```python
from build123d import *

# Parameters (mm, degrees)
F0_R     = 1.984375
F1_DEPTH = 9.525
F3_R     = 3.175
F4_DEPTH = 4.7625
F6_DEPTH = 3.96875


with BuildPart() as f1:
    # F0 (on Front) → F1 (new body)
    with BuildSketch(Plane.XZ):
        Circle(F0_R)
    extrude(amount=F1_DEPTH)

    # F3 (on face) → F4 (join)
    with BuildSketch(Plane.XZ.offset(9.525)):
        Circle(F3_R)
    extrude(amount=F4_DEPTH)

    # F5 (on face) → F6 (cut)
    with BuildSketch(Plane.XZ.offset(14.2875)):
        Polygon((1.984375, 1.145679), (0, 2.291359), (-1.984375, 1.145679), (-1.984375, -1.145679), (0, -2.291359), (1.984375, -1.145679), align=None)
    extrude(amount=-F6_DEPTH, mode=Mode.SUBTRACT)


solid = f1.part
```
Work out the finished part from the listing and answer in its coordinate system (mm). A direction names the side the tool comes from. Round coordinates to 2 decimals unless told otherwise and drop trailing zeros. Write each loop counter-clockwise with the first axis right and the second up, starting at its lowest first coordinate (ties: lowest second). Pieces come first, ordered by that corner, then holes.
1) A cutting plane is placed at C-C on y = -5.75. Determine the outline of the cut face in (x, z), and give its area (3 significant figures).
2) A cutting plane is placed at A-A on z = 0. Determine the outline of the cut face in (x, y) (1 decimal), and give its area (3 significant figures).
3) A cutting plane is placed at B-B on x = 1.75. Determine the outline of the cut face in (y, z) (1 decimal).
4) Which of the six approach directions +Z, -Z, +X, -X, +Y, -Y give full straight-line access (tool end or side, diameter ignored) to faces 4 (the face through (0.978, -12.331, -1.727)), 5 (the face through (1, -9.525, -2)), 6 (the face through (0, 0, 0))?
5) Consider probe 1 along Y at (x, z) = (0.25, -1); probe 2 along X at (y, z) = (-12.75, 0.75); probe 3 along Z at (x, y) = (0.5, -11). Determine where each line is inside the solid, lowest interval first.
6) A cutting plane is placed at D-D on x = -3. Determine the outline of the cut face in (y, z) (1 decimal), and give its area (3 significant figures).
7) Determine the mould class of faces 1 (the face through (1.984, -12, 0)), 2 (the face through (1, -14.288, -2)), 3 (the face through (-0.69, -11.87, -3.1)) for opening direction Z: pulls with the +Z half, pulls with the -Z half, needs draft (parallel to the pull), parting line crosses it, or undercut.
8) Flat-ended cylindrical pins translate along their axes: P1, Ø2, axis at y = -6, z = -0.5, coming from the -X side; P2, Ø1.5, axis at y = -2.5, z = 2, coming from the -X side; P3, Ø2, axis at x = -1.5, y = -4, coming from the -Z side; P4, Ø2, axis at x = -1.5, z = 0, coming from the -Y side. Find the tip coordinate at first contact, or state that the pin passes through.
Entries:
1. outline: circle Ø3.97 at (0, 0)
1. area: 12.4 mm2
2. outline: (-3.2, -14.3) - (-2, -14.3) - (-2, -10.3) - (2, -10.3) - (2, -14.3) - (3.2, -14.3) - (3.2, -9.5) - (2, -9.5) - (2, 0) - (-2, 0) - (-2, -9.5) - (-3.2, -9.5) - close
2. area: 52.3 mm2
3. outline: (-14.3, -2.6) - (-9.5, -2.6) - (-9.5, -0.9) - (0, -0.9) - (0, 0.9) - (-9.5, 0.9) - (-9.5, 2.6) - (-14.3, 2.6) - (-14.3, 1.3) - (-10.3, 1.3) - (-10.3, -1.3) - (-14.3, -1.3) - close
4. face 4: -Y
4. face 5: +Y
4. face 6: +Z, -Z, +X, -X, +Y
5. probe 1: y = -10.32 to 0
5. probe 2: x = -3.09 to -1.98, 1.98 to 3.09
5. probe 3: z = -3.14 to -2, 2 to 3.14
6. outline: (-14.3, -1) - (-9.5, -1) - (-9.5, 1) - (-14.3, 1) - close
6. area: 9.90 mm2
7. face 1: undercut
7. face 2: needs draft
7. face 3: parting line crosses it
8. P1: stops at x = -1.98
8. P2: stops at x = -1.54
8. P3: stops at z = -1.92
8. P4: stops at y = -14.29
